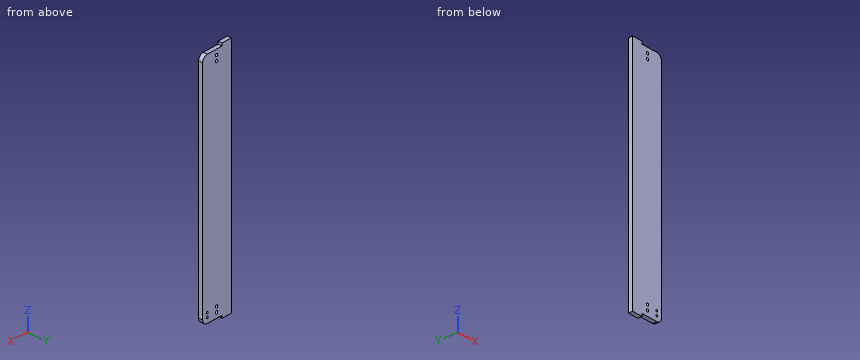
Autodesk Inventor part; units mm, degrees
ref_plane "YZ Plane" through (0, 0, 0) normal (1, 0, 0) x (0, 1, 0)
ref_plane "XZ Plane" through (0, 0, 0) normal (0, 1, 0) x (-1, 0, 0)
ref_plane "XY Plane" through (0, 0, 0) normal (0, 0, 1) x (1, 0, 0)
sketch "Sketch1" plane through (0, 0, 0) normal (0, 1, 0) x (-1, 0, 0)
  line L0 (0, 0) -> (62, 0)
  line L1 (62, 0) -> (62, -450)
  line L2 (62, -450) -> (0, -450)
  line L3 (0, -450) -> (0, 0)
  dimension "d0" = 62
  dimension "d1" = 450
extrude "Extrusion1" add sketch "Sketch1" along normal blind 8
fillet "Fillet1" radius 10 2 edges at (0, 4, 0) (0, 4, -450)
sketch "Sketch3" plane through (0, 8, 0) normal (0, 1, 0) x (1, 0, 0)
  point P0 (0, 0)
sketch "Sketch4" plane through (0, 8, 0) normal (0, 1, 0) x (1, 0, 0)
  circle A0 centre (-10, 440) radius 2
  circle A1 centre (-10, 432) radius 2
  line L0 (0, 10) -> (0, 440)
  line L1 (-10, 450) -> (-62, 450)
  point P0 (0, 0)
  dimension "d25" = 10
  dimension "d26" = 10
  dimension "d27" = 4
  dimension "d28" = 4
  dimension "d29" = 10
  dimension "d30" = 8
hole "Hole2" at (-10, 8, -432) at (-10, 8, -440) direction (0, -1, 0) diameter 4 end through all
sketch "Sketch5" plane through (0, 8, 0) normal (0, 1, 0) x (1, 0, 0)
  point P0 (0, 0)
sketch "Sketch6" plane through (0, 8, 0) normal (0, 1, 0) x (1, 0, 0)
  circle A0 centre (-30, 20) radius 2.6
  circle A1 centre (-30, 10) radius 2.6
  line L0 (-62, 0) -> (-10, 0)
  line L1 (-62, 450) -> (-62, 0)
  line L2 (-101.8296, 225) -> (129.7674, 225) construction
  circle A2 centre (-30, 430) radius 2.6
  circle A3 centre (-30, 440) radius 2.6
  point P0 (0, 0)
  point P1 (-10, 450)
  dimension "d38" = 5.2
  dimension "d39" = 5.2
  dimension "d40" = 20
  dimension "d41" = 10
  dimension "d42" = 32
  dimension "d43" = 32
  dimension "d44" = 225
hole "Hole3" at (-30, 8, -20) at (-30, 8, -10) at (-30, 8, -440) at (-30, 8, -430) direction (0, -1, 0) diameter 5.2 end through all
sketch "Sketch7" plane through (0, 8, 0) normal (0, 1, 0) x (1, 0, 0)
  line L0 (-62, 450) -> (-62, 0)
  line L1 (-62, 0) -> (-42, 0)
  line L2 (-42, 0) -> (-42, -5)
  line L3 (-42, -5) -> (-62, -5)
  line L4 (-62, -5) -> (-62, 0)
  line L5 (-62, 450) -> (-42, 450)
  line L6 (-42, 450) -> (-42, 455)
  line L7 (-42, 455) -> (-62, 455)
  line L8 (-62, 455) -> (-62, 450)
  point P0 (0, 0)
  dimension "d52" = 20
  dimension "d53" = 5
  dimension "d54" = 20
  dimension "d55" = 5
extrude "Extrusion2" add sketch "Sketch7" against normal blind 8
equation "\"d31\" = d28"
properties part number "X_Kettenhalter"
The model under review builds one solid part; all positions refer to its coordinate system, in mm. Round coordinates to 2 decimals unless told otherwise and drop trailing zeros. Loops run counter-clockwise (first coordinate to the right, second up) from the corner with the lowest first, then second, coordinate; pieces in that order, holes last.
Item 1: Clearance check with flat-ended pins moving along their axes: pin 1 Ø3.5 at (x, z) = (-10, -440) entering from +Y; pin 2 Ø2 at (x, y) = (-15.5, 2.5) entering from +Z; pin 3 Ø2.5 at (y, z) = (4, -453.5) entering from +X; pin 4 Ø1 at (x, y) = (-7, 6.5) entering from +Z. State where each tip first meets the part, or that it passes through.
Determined:
pin 1: passes through
pin 2: stops at z = 0
pin 3: stops at x = -42
pin 4: stops at z = -0.32
Item 2: Take a section at A-A (y = 1.75). Write out the cut boundary in (x, z).
Determined:
outline: (-62, -455) - (-42, -455) - (-42, -450) - (-10, -450) arc R10 ccw to (0, -440) - (0, -10) arc R10 ccw to (-10, 0) - (-42, 0) - (-42, 5) - (-62, 5) - close; hole circle Ø5.2 at (-30, -440); hole circle Ø5.2 at (-30, -430); hole circle Ø5.2 at (-30, -20); hole circle Ø5.2 at (-30, -10); hole circle Ø4 at (-10, -440); hole circle Ø4 at (-10, -432)
Item 3: For line 1 (Z direction, x = -10, y = 2.75); line 2 (Z direction, x = -30, y = 6.5); line 3 (X direction, y = 3.5, z = -440), list the stretches that pass through material, from the lowest coordinate up.
Determined:
line 1: z = -450 to -442, -438 to -434, -430 to 0
line 2: z = -450 to -442.6, -437.4 to -432.6, -427.4 to -22.6, -17.4 to -12.6, -7.4 to 0
line 3: x = -62 to -32.6, -27.4 to -12, -8 to 0
